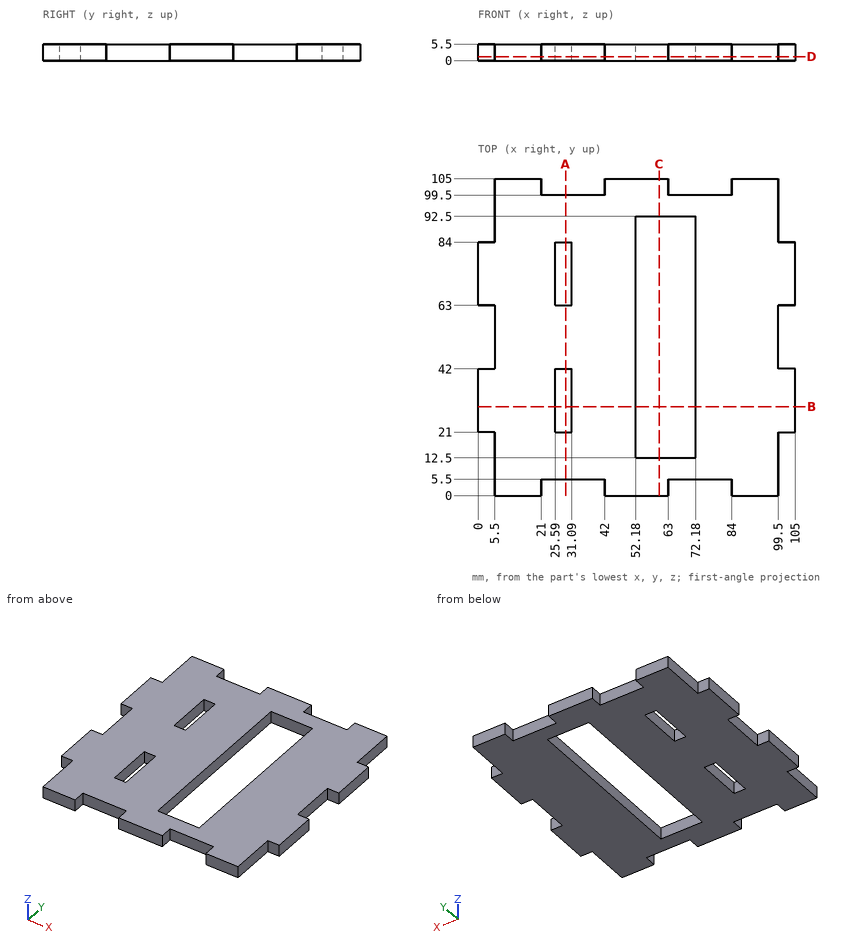
The figure shows three views and two pictorial views of one solid part (mm, origin at its lowest corner). Answer the questions. Give positions to 0.01 mm unless a question says otherwise; leave off trailing zeros. Write each loop counter-clockwise with the first axis right and the second up, starting at its lowest first coordinate (ties: lowest second). Pieces come first, ordered by that corner, then holes. Notation, with made-up numbers: (54.25, 19.5) - (73.25, 19.5) arc R20 cw to (73.25, 35.5) - close; hole circle Ø4 at (44.25, 63.5). An arc over 180 degrees is marked (long way). Return JSON: item names as keys, results as strings.
Q1. A cutting plane is placed at D-D, the plane z = 1.35. Count the separate pieces of the cut face and the enclosed holes in it, and give its area (3 significant figures).
Reply:
{"separate pieces": "1", "enclosed holes": "3", "area": "8,040 mm²"}
Q2. A cutting plane is placed at B-B, the plane y = 29.5. Determine the outline of the cut face in (x, z).
Reply:
{"outline": "(0, 0) - (25.59, 0) - (25.59, 5.5) - (0, 5.5) - close; (31.09, 0) - (52.18, 0) - (52.18, 5.5) - (31.09, 5.5) - close; (72.18, 0) - (105, 0) - (105, 5.5) - (72.18, 5.5) - close"}
Q3. Consider line 1 along X through (y, z) = (30.5, 4.2); line 2 along X through (y, z) = (101, 4.8); line 3 along X through (y, z) = (48, 0.5). Determine where each line is inside the solid, lowest interval first. Write a range as [from, to].
Reply:
{"line 1": "[0, 25.59], [31.09, 52.18], [72.18, 105]", "line 2": "[5.5, 21], [42, 63], [84, 99.5]", "line 3": "[5.5, 52.18], [72.18, 99.5]"}
Q4. A cutting plane is placed at A-A, the plane x = 29. Determine the outline of the cut face in (y, z), and give its area (3 significant figures).
Reply:
{"outline": "(5.5, 0) - (21, 0) - (21, 5.5) - (5.5, 5.5) - close; (42, 0) - (63, 0) - (63, 5.5) - (42, 5.5) - close; (84, 0) - (99.5, 0) - (99.5, 5.5) - (84, 5.5) - close", "area": "286 mm²"}
Q5. Given P1, Ø1.6, axis at y = 3, z = 2.5, coming from the -X side; P2, Ø3, axis at y = 102, z = 2, coming from the +X side; P3, Ø4, axis at x = 70, y = 20.5, coming from the +Z side; P4, Ø3, axis at x = 3.5, z = 2, coming from the +Y side, each flat-ended and moving along its own axis, determine where each tip first touches the part or whether it passes through.
Reply:
{"P1": "x = 5.5", "P2": "x = 99.5", "P3": "through", "P4": "y = 84"}
Q6. A cutting plane is placed at C-C, the plane x = 60. Determine the outline of the cut face in (y, z), and give its area (4 significant figures).
Reply:
{"outline": "(0, 0) - (12.5, 0) - (12.5, 5.5) - (0, 5.5) - close; (92.5, 0) - (105, 0) - (105, 5.5) - (92.5, 5.5) - close", "area": "137.5 mm²"}
